Geometry check sheet. Reference: drawing and pictorial views, mm from the part's lowest x, y, z. Give positions to 0.01 mm unless a question says otherwise; leave off trailing zeros. Order: outer loops, then holes, each group sorted by start corner. A loop starts at its lowest first (then second) coordinate and runs counter-clockwise, first axis right, second up. Notation, with made-up numbers: (69.25, -11.5) - (116.25, -11.5) arc R20 ccw to (116.25, 11.5) - close; hole circle Ø11 at (-5.75, -36). An arc over 180 degrees is marked (long way). Answer in a Markdown table with one row per item.
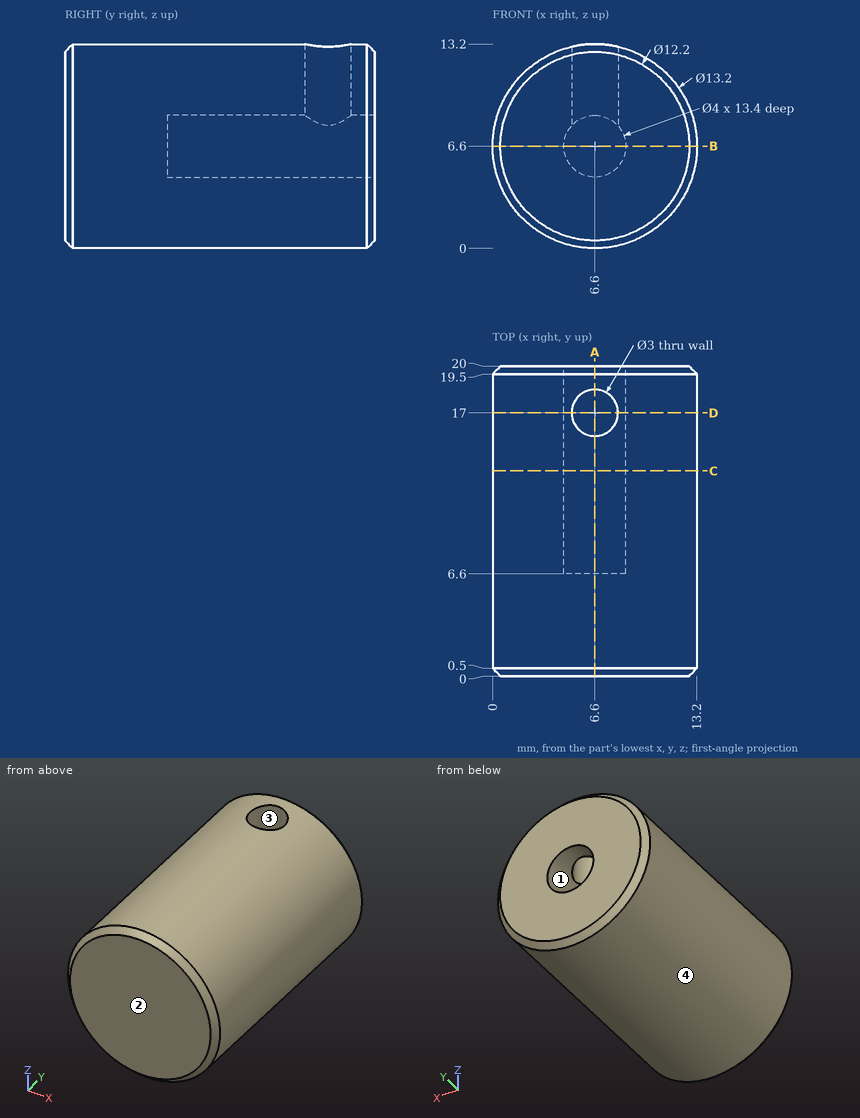
(1) Cross-section at D-D, the plane y = 17. Record the cut outline in (x, z).
Geometry says:
| item | result |
|---|---|
| outline | (5.1, 7.92) - (5.1, 13.03) arc R6.6 ccw (long way) to (8.1, 13.03) - (8.1, 7.92) arc R2 cw (long way) to start |
(2) Cross-section at A-A, the plane x = 6.6. Record the cut outline in (y, z), then the cut area to 3 significant figures.
Geometry says:
| item | result |
|---|---|
| outline | (0, 0.5) - (0.5, 0) - (19.5, 0) - (20, 0.5) - (20, 4.6) - (6.6, 4.6) - (6.6, 8.6) - (15.5, 8.6) - (15.5, 13.2) - (0.5, 13.2) - (0, 12.7) - close; (18.5, 8.6) - (20, 8.6) - (20, 12.7) - (19.5, 13.2) - (18.5, 13.2) - close |
| area | 196 mm² |
(3) Thickness scan on L1, parallel to X at y = 17, z = 6.6; L2, parallel to Y at x = 6.5, z = 10.5; L3, parallel to Z at x = 7.25, y = 10.25. Record the ranges inside material, lowest first.
Geometry says:
| item | result |
|---|---|
| L1 | 0 to 4.6, 8.6 to 13.2 |
| L2 | 0 to 15.5, 18.5 to 20 |
| L3 | 0.03 to 4.71, 8.49 to 13.17 |
(4) Mould release check, pull along X, two halves, no side actions. Record for the marked faces 1, 2, 3 and 4: pulls with the +X half, pulls with the -X half, needs draft (parallel to the pull), parting line crosses it, or undercut.
Geometry says:
| item | result |
|---|---|
| face 1 | undercut |
| face 2 | needs draft |
| face 3 | undercut |
| face 4 | parting line crosses it |
(5) Cross-section at C-C, the plane y = 13.25. Record the cut outline in (x, z), then the cut area to 3 significant figures.
Geometry says:
| item | result |
|---|---|
| outline | circle Ø13.2 at (6.6, 6.6); hole circle Ø4 at (6.6, 6.6) |
| area | 124 mm² |
(6) Cross-section at B-B, the plane z = 6.6. Record the cut outline in (x, y).
Geometry says:
| item | result |
|---|---|
| outline | (0, 0.5) - (0.5, 0) - (12.7, 0) - (13.2, 0.5) - (13.2, 19.5) - (12.7, 20) - (8.6, 20) - (8.6, 6.6) - (4.6, 6.6) - (4.6, 20) - (0.5, 20) - (0, 19.5) - close |
(7) Gauge pin test, flat ends, axial feed: P1, Ø2, axis at y = 3.5, z = 9.5, coming from the +X side; P2, Ø5, axis at y = 12.5, z = 10, coming from the -X side. Record the tip position at first contact, or that the pin passes through.
Geometry says:
| item | result |
|---|---|
| P1 | x = 12.92 |
| P2 | x = 0.06 |
